```python
from build123d import *

# Parameters (mm, degrees)
F0_W      = 90
F0_H      = 22
F1_DEPTH  = 10
F3_DEPTH  = 5
F4_R      = 2
F5_W      = 90
F5_H      = 22
F6_DEPTH  = 10
F8_DEPTH  = 10
F9_R      = 2
F11_DEPTH = 45
F13_DEPTH = 45
F14_R     = 2
F15_W     = 50
F15_H     = 22
F16_DEPTH = 10
F17_R     = 5
F18_DEPTH = 25
F18_TAPER = 3
F20_R     = 3
F21_DEPTH = 90
F22_R     = 2.5
F23_DEPTH = 3.1
F23_TAPER = -3
F24_R     = 2.5
F25_DEPTH = 3.1
F25_TAPER = -3


with BuildPart() as f1:
    # F0 (on Top) → F1 (new body)
    with BuildSketch(Plane.XY):
        with Locations((0, -55.5313304067)):
            Rectangle(F0_W, F0_H)
    extrude(amount=F1_DEPTH)

    # F2 (on face) → F3 (cut)
    with BuildSketch(Plane(origin=(0, 0, 0), x_dir=(1, 0, 0), z_dir=(0, 0, -1))):
        Polygon((-39.5, 44.5313304067), (0, 44.5313304067), (39.5, 44.5313304067), (39.19890013, 61.7813304067), (-39.19890013, 61.7813304067), align=None)
    extrude(amount=-F3_DEPTH, mode=Mode.SUBTRACT)

    # F4
    f4_edges = [f1.edges().sort_by_distance(p)[0] for p in [
        (-39.1989, -61.78133, 2.5),
        (39.1989, -61.78133, 2.5),
    ]]
    fillet(f4_edges, radius=F4_R)

    # F5 (on face) → F6 (join)
    with BuildSketch(Plane(origin=(0, 0, 0), x_dir=(1, 0, 0), z_dir=(0, 0, -1))):
        with Locations((0, 55.5313304067)):
            Rectangle(F5_W, F5_H)
    extrude(amount=F6_DEPTH)

    # F7 (on face) → F8 (cut)
    with BuildSketch(Plane(origin=(0, 0, -10), x_dir=(1, 0, 0), z_dir=(0, 0, -1))):
        Polygon((-20, 44.5313304067), (0, 44.5313304067), (20, 44.5313304067), (19.8167218183, 55.0313304067), (-19.8167218183, 55.0313304067), align=None)
        Polygon((19.8167218183, 55.0313304067), (20, 44.5313304067), (20, 55.0313304067), align=None)
        Polygon((-20, 55.0313304067), (-20, 44.5313304067), (-19.8167218183, 55.0313304067), align=None)
    extrude(amount=-F8_DEPTH, mode=Mode.SUBTRACT)

    # F9
    f9_edges = [f1.edges().sort_by_distance(p)[0] for p in [
        (-20, -55.03133, -5),
        (20, -55.03133, -5),
    ]]
    fillet(f9_edges, radius=F9_R)

    # F10 (on face) → F11 (join)
    with BuildSketch(Plane(origin=(0, 0, -10), x_dir=(1, 0, 0), z_dir=(0, 0, -1))):
        Polygon((-25, 44.5313304067), (0, 44.5313304067), (25, 44.5313304067), (25, 66.5313304067), (-25, 66.5313304067), align=None)
    extrude(amount=F11_DEPTH)

    # F12 (on face) → F13 (cut)
    with BuildSketch(Plane(origin=(0, 0, -55), x_dir=(1, 0, 0), z_dir=(0, 0, -1))):
        Polygon((-17.5, 44.5313304067), (0, 44.5313304067), (17.5, 44.5313304067), (17.3603594806, 52.5313304067), (-17.3603594806, 52.5313304067), align=None)
    extrude(amount=-F13_DEPTH, mode=Mode.SUBTRACT)

    # F14
    f14_edges = [f1.edges().sort_by_distance(p)[0] for p in [
        (-17.360359, -52.53133, -32.5),
        (17.360359, -52.53133, -32.5),
    ]]
    fillet(f14_edges, radius=F14_R)

    # F15 (on face) → F16 (join)
    with BuildSketch(Plane(origin=(0, 0, -55), x_dir=(1, 0, 0), z_dir=(0, 0, -1))):
        with Locations((0, 55.5313304067)):
            Rectangle(F15_W, F15_H)
    extrude(amount=F16_DEPTH)

    # F17 (on face) → F18 (cut)
    with BuildSketch(Plane(origin=(0, 0, -65), x_dir=(1, 0, 0), z_dir=(0, 0, -1))):
        with Locations((0, 44.5313304067)):
            Circle(F17_R)
    extrude(amount=-F18_DEPTH, taper=F18_TAPER, mode=Mode.SUBTRACT)

    # F20 (on face) → F21 (cut)
    with BuildSketch(Plane.XY.offset(10)):
        with Locations((22.7543748915, -44.5189550519)):
            Circle(F20_R)
        with Locations((-22.8854361922, -44.5189550519)):
            Circle(F20_R)
    extrude(amount=-F21_DEPTH, mode=Mode.SUBTRACT)

    # F22 (on face) → F23 (cut)
    with BuildSketch(Plane(origin=(0, -44.5313304067, 0), x_dir=(-1, 0, 0), z_dir=(0, 1, 0))):
        with Locations((-15.0013593957, -60.537815094)):
            Circle(F22_R)
        with Locations((15.0013593957, -60.537815094)):
            Circle(F22_R)
    extrude(amount=-F23_DEPTH, taper=F23_TAPER, mode=Mode.SUBTRACT)

    # F24 (on face) → F25 (cut)
    with BuildSketch(Plane(origin=(0, -44.5313304067, 0), x_dir=(-1, 0, 0), z_dir=(0, 1, 0))):
        with Locations((-42, 7.0607517846)):
            Circle(F24_R)
        with Locations((42, 7.0607517846)):
            Circle(F24_R)
    extrude(amount=-F25_DEPTH, taper=F25_TAPER, mode=Mode.SUBTRACT)


solid = f1.part
```
Can you work these out from the model? Positions are in its coordinate system, mm. A direction names the side the tool comes from. Round coordinates to 2 decimals unless told otherwise and drop trailing zeros. Loops run counter-clockwise (first coordinate to the right, second up) from the corner with the lowest first, then second, coordinate; pieces in that order, holes last. Notation, with made-up numbers: (83.25, 77) -> (119.25, 77) arc R19 ccw to (119.25, 109) -> close; hole circle Ø8 at (55.5, 18.25). An arc over 180 degrees is marked (long way). One line per item, written item: value. Start each with the question number.
1. If I drill on probe 1 along X at (y, z) = (-49, -7.5); probe 2 along Z at (x, y) = (29.5, -50); probe 3 along Z at (x, y) = (-11.5, -46.25), over which ranges is the centre line in solid material (lowest first)?
2. For faces 1 (the flat face through (25, -56, -37)), 2 (the conical face through (44.05, -46.1, 5.49)), 3 (the flat face through (20, -49, -5)), which set-ups out of +Z, -Z, +X, -X, +Y, -Y let a thin tool reach every point of the face, with its end or its side?
3. If we section it at B-B, the plane x = 29.5: Write out the boundary of the cut face in (y, z).
4. If we section it at C-C, the plane y = -63: Write out the boundary of the cut face in (x, z).
5. If we section it at A-A, the plane z = -4.5: Write out the boundary of the cut face in (x, y), then the cut area to 3 significant figures.
6. If we mould it in two halves opening along Y, with no side actions, what happens to faces 4 (the cylindrical face through (-19.4, -54.46, -4.93)), 5 (the flat face through (35, -56, -10)), 6 (the conical face through (-17.464, -46.103, -59.762)), 7 (the conical face through (-39.95, -46.1, 5.49))? For each: pulls with the +Y half, pulls with the -Y half, needs draft (parallel to the pull), parting line crosses it, or undercut.
7. If we section it at D-D, the plane y = -57: Write out the boundary of the cut face in (x, z), then the cut area to 3 significant figures.
8. For pin 1 (9 mm diameter, centred on x = -6.5, z = -36.5, fed in from +Y); pin 2 (10 mm diameter, centred on y = -49, z = -44.5, fed in from -X); pin 3 (6 mm diameter, centred on x = -39.5, y = -56, fed in from -Z), each with a flat end and sliding along its axis, tell me the tip position at first contact or that it passes through.
Calculated:
1. probe 1: x = -45 to -20, 20 to 45
1. probe 2: z = -10 to 0, 5 to 10
1. probe 3: z = -65 to -55, 5 to 10
2. face 1: -Z, +X, +Y, -Y
2. face 2: none
2. face 3: +Y
3. outline: (-66.53, -10) -> (-44.53, -10) -> (-44.53, 0) -> (-61.78, 0) -> (-61.78, 5) -> (-44.53, 5) -> (-44.53, 10) -> (-66.53, 10) -> close
4. outline: (-45, -10) -> (-25, -10) -> (-25, -65) -> (25, -65) -> (25, -10) -> (45, -10) -> (45, 10) -> (-45, 10) -> close
5. outline: (-45, -66.53) -> (45, -66.53) -> (45, -44.53) -> (25.75, -44.53) arc R3 cw to (20, -45.71) -> (20, -53.03) arc R2 cw to (18, -55.03) -> (-18, -55.03) arc R2 cw to (-20, -53.03) -> (-20, -45.34) arc R3 cw to (-25.89, -44.53) -> (-45, -44.53) -> close
5. area: 1,530 mm²
6. face 4: pulls with the +Y half
6. face 5: needs draft
6. face 6: undercut
6. face 7: undercut
7. outline: (-45, -10) -> (-25, -10) -> (-25, -65) -> (25, -65) -> (25, -10) -> (45, -10) -> (45, 10) -> (-45, 10) -> close; hole (-39.28, 0) -> (39.28, 0) -> (39.28, 5) -> (-39.28, 5) -> close
7. area: 4,160 mm²
8. pin 1: stops at y = -52.53
8. pin 2: stops at x = -25
8. pin 3: stops at z = -10
